Verification items for the finished model (mm, model axes). Face numbers are marked on the shaded views. Round coordinates to 2 decimals unless told otherwise and drop trailing zeros. Loops run counter-clockwise (first coordinate to the right, second up) from the corner with the lowest first, then second, coordinate; pieces in that order, holes last. Notation, with made-up numbers: (-36.75, 58.25) -> (-17.75, 58.25) arc R30 ccw to (-17.75, 88.25) -> close; hole circle Ø5 at (19, 36). An arc over 180 degrees is marked (long way). Use CSV: the item, a comma, the result in double quotes. Start each with the question number.
```python
from build123d import *

# Parameters (mm, degrees)
BOSS_EXTRUDE1_DEPTH = 3.175
EXTRUDE_THIN1_START = -6.1722
EXTRUDE_THIN1_DEPTH = 6.1722
SKETCH5_R           = 1.475
BOSS_EXTRUDE2_DEPTH = 5
SKETCH6_R           = 1.55
CUT_EXTRUDE1_DEPTH  = 213.890793601
CHAMFER1_SIZE       = 0.508
SKETCH7_R           = 2.5
BOSS_EXTRUDE3_DEPTH = 0.254


with BuildPart() as part:
    # Sketch1 → Boss-Extrude1 (new body)
    with BuildSketch(Plane.ZY.offset(-35.1028)):
        with BuildLine():
            Line((-114.3, 38.1), (-114.3, -38.1))
            Line((-114.3, -38.1), (-184.15, -38.1))
            ThreePointArc((-184.15, -38.1), (-188.640128061, -36.240128061), (-190.5, -31.75))
            Line((-190.5, -31.75), (-190.5, 31.75))
            ThreePointArc((-190.5, 31.75), (-188.640128061, 36.240128061), (-184.15, 38.1))
            Line((-184.15, 38.1), (-114.3, 38.1))
        make_face()
    extrude(amount=BOSS_EXTRUDE1_DEPTH)

    # Sketch4 → Extrude-Thin1 (add)
    with BuildSketch(Plane.ZY.offset(-31.9278).offset(EXTRUDE_THIN1_START)):
        with BuildLine():
            Line((-114.3, 38.1), (-184.15, 38.1))
            ThreePointArc((-184.15, 38.1), (-188.640128061, 36.240128061), (-190.5, 31.75))
            Line((-190.5, 31.75), (-190.5, -31.75))
            ThreePointArc((-190.5, -31.75), (-188.640128061, -36.240128061), (-184.15, -38.1))
            Line((-184.15, -38.1), (-114.3, -38.1))
            Line((-114.3, -38.1), (-114.3, -40.64))
            Line((-114.3, -40.64), (-184.15, -40.64))
            ThreePointArc((-184.15, -40.64), (-190.436179285, -38.036179285), (-193.04, -31.75))
            Line((-193.04, -31.75), (-193.04, 31.75))
            ThreePointArc((-193.04, 31.75), (-190.436179285, 38.036179285), (-184.15, 40.64))
            Line((-184.15, 40.64), (-114.3, 40.64))
            Line((-114.3, 40.64), (-114.3, 38.1))
        make_face()
    extrude(amount=EXTRUDE_THIN1_DEPTH)

    # Sketch5 → Boss-Extrude2 (add)
    with BuildSketch(Plane.ZY.offset(-31.9278)):
        with Locations(Location((-186.69, 33.075, 0), (0, 0, 180))):
            Circle(SKETCH5_R)
        with Locations(Location((-120.65, 33.075, 0), (0, 0, 180))):
            Circle(SKETCH5_R)
        with Locations(Location((-120.65, -33.075, 0), (0, 0, 180))):
            Circle(SKETCH5_R)
        with Locations(Location((-186.69, -33.075, 0), (0, 0, 180))):
            Circle(SKETCH5_R)
    extrude(amount=BOSS_EXTRUDE2_DEPTH)

    # Sketch6 → Cut-Extrude1 (cut, through all)
    with BuildSketch(Plane(origin=(0, 40.64, 0), x_dir=(1, 0, 0), z_dir=(0, 1, 0))):
        with Locations((32.9698, 173.99)):
            Circle(SKETCH6_R)
        with Locations((32.9698, 133.35)):
            Circle(SKETCH6_R)
    extrude(amount=-CUT_EXTRUDE1_DEPTH, mode=Mode.SUBTRACT)

    # Chamfer1
    chamfer1_edges = [part.edges().sort_by_distance(p)[0] for p in [
        (26.9278, -33.075, -185.215),
        (26.9278, -33.075, -119.175),
        (26.9278, 33.075, -119.175),
        (26.9278, 33.075, -185.215),
    ]]
    chamfer(chamfer1_edges, length=CHAMFER1_SIZE)

    # Sketch7 → Boss-Extrude3 (add)
    with BuildSketch(Plane.ZY.offset(-31.9278)):
        with Locations(Location((-186.69, 33.075, 0), (0, 0, 180))):
            Circle(SKETCH7_R)
        with Locations(Location((-120.65, 33.075, 0), (0, 0, 180))):
            Circle(SKETCH7_R)
        with Locations(Location((-120.65, -33.075, 0), (0, 0, 180))):
            Circle(SKETCH7_R)
        with Locations(Location((-186.69, -33.075, 0), (0, 0, 180))):
            Circle(SKETCH7_R)
    extrude(amount=BOSS_EXTRUDE3_DEPTH)


solid = part.part
```
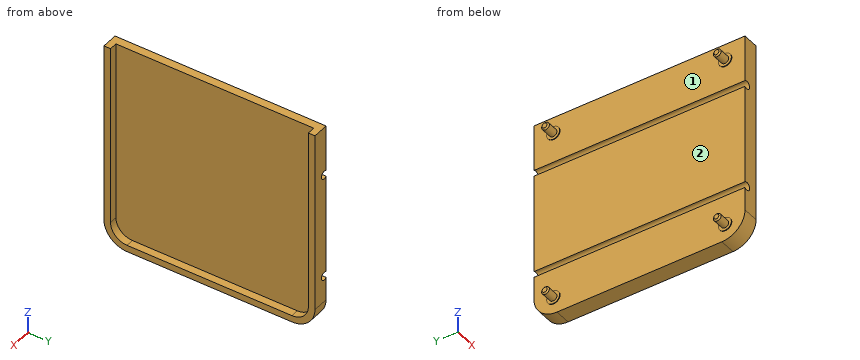
Q1. Cross-section at B-B (x = 36.5). Record the boundary of the cut face in (y, z), and give its area (3 significant figures).
Q2. Depth check by flat-ended pin: pin 1 Ø14.5 at (y, z) = (17, -181) entering from -X; pin 2 Ø2.5 at (x, z) = (32.97, -173.99) entering from -Y (3 decimals); pin 3 Ø4 at (y, z) = (7.5, -145) entering from +X; pin 4 Ø0.9 at (x, y) = (37, -5.5) entering from +Z. Enter the tip coordinate at first touch or a pass-through.
Q3. Release check for a two-part mould opening along Y. For the marked faces 1 and 2 record: +Y half, -Y half, draft (parallel to the pull), parting line (faces both ways), or undercut.
Q4. Cross-section at D-D (z = -173.99). Record the boundary of the cut face in (x, y), and give its area (3 significant figures).
Q5. Cross-section at C-C (y = -4). Record the boundary of the cut face in (x, z), and give its area (3 significant figures).
Q6. Thickness scan on L1, parallel to Y at x = 28.25, z = -186.5; L2, parallel to Z at x = 33.75, y = 16; L3, parallel to Y at x = 35.5, z = -161. Record the ranges inside material, lowest first. Write a range as from..to.
Q7. Cross-section at A-A (z = -120.65). Record the boundary of the cut face in (x, y) (3 decimals).
Answer list:
1,outline,"(-40.64, -184.15) arc R8.89 ccw to (-31.75, -193.04) -> (31.75, -193.04) arc R8.89 ccw to (40.64, -184.15) -> (40.64, -114.3) -> (38.1, -114.3) -> (38.1, -184.15) arc R6.35 cw to (31.75, -190.5) -> (-31.75, -190.5) arc R6.35 cw to (-38.1, -184.15) -> (-38.1, -114.3) -> (-40.64, -114.3) -> close"
1,area,"577 mm2"
2,pin 1,"stops at x = 31.93"
2,pin 2,"passes through"
2,pin 3,"stops at x = 35.1"
2,pin 4,"stops at z = -190.5"
3,face 1,"undercut"
3,face 2,"draft"
4,outline,"(34.52, -40.64) -> (38.1, -40.64) -> (38.1, -38.1) -> (35.1, -38.1) -> (35.1, 38.1) -> (38.1, 38.1) -> (38.1, 40.64) -> (34.52, 40.64) -> close"
4,area,"62.6 mm2"
5,outline,"(31.93, -193.04) -> (38.1, -193.04) -> (38.1, -190.5) -> (35.1, -190.5) -> (35.1, -114.3) -> (31.93, -114.3) -> (31.93, -132.2) arc R1.55 cw (long way) to (31.93, -134.5) -> (31.93, -172.84) arc R1.55 cw (long way) to (31.93, -175.14) -> close"
5,area,"244 mm2"
6,L1,"y = -34.54..-31.61, 31.61..34.54"
6,L2,"z = -193.04..-175.33, -172.65..-134.69, -132.01..-114.3"
6,L3,"y = -40.64..-38.1, 38.1..40.64"
7,outline,"(26.928, -34.042) -> (27.436, -34.55) -> (31.674, -34.55) -> (31.674, -35.575) -> (31.928, -35.575) -> (31.928, -40.64) -> (38.1, -40.64) -> (38.1, -38.1) -> (35.103, -38.1) -> (35.103, 38.1) -> (38.1, 38.1) -> (38.1, 40.64) -> (31.928, 40.64) -> (31.928, 35.575) -> (31.674, 35.575) -> (31.674, 34.55) -> (27.436, 34.55) -> (26.928, 34.042) -> (26.928, 32.108) -> (27.436, 31.6) -> (31.674, 31.6) -> (31.674, 30.575) -> (31.928, 30.575) -> (31.928, -30.575) -> (31.674, -30.575) -> (31.674, -31.6) -> (27.436, -31.6) -> (26.928, -32.108) -> close"
